Autodesk Fusion 360 part; units mm, degrees
sketch "Sketch1" plane through (0, 0, 0) normal (0, 0, 1) x (1, 0, 0)
  line L0 (0, 57.15) -> (0, 0)
  line L1 (101.6, 57.15) -> (130.175, 57.15)
  line L2 (130.175, 57.15) -> (130.175, 25.4)
  line L3 (130.175, 25.4) -> (101.6, 25.4)
  line L4 (101.6, 25.4) -> (101.6, 57.15)
  line L5 (115.8875, 25.4) -> (115.8875, 0) construction
  line L6 (106.3625, 25.4) -> (106.3625, 0)
  line L7 (125.4125, 25.4) -> (125.4125, 0)
  line L8 (12.7, 57.15) -> (12.7, 12.7)
  line L9 (12.7, 12.7) -> (28.575, 12.7)
  line L10 (28.575, 12.7) -> (28.575, 57.15)
  line L11 (14.2875, 12.7) -> (14.2875, 0)
  line L12 (26.9875, 12.7) -> (26.9875, 0)
  line L13 (12.7, 57.15) -> (28.575, 57.15)
  line L14 (14.2875, 0) -> (26.9875, 0)
  line L15 (106.3625, 0) -> (125.4125, 0)
  line L16 (36.5125, 0) -> (49.2125, 0)
  line L17 (34.925, 57.15) -> (50.8, 57.15)
  line L18 (49.2125, 12.7) -> (49.2125, 0)
  line L19 (34.925, 57.15) -> (34.925, 12.7)
  line L20 (36.5125, 12.7) -> (36.5125, 0)
  line L21 (34.925, 12.7) -> (50.8, 12.7)
  line L22 (50.8, 12.7) -> (50.8, 57.15)
  line L23 (58.7375, 0) -> (71.4375, 0)
  line L24 (57.15, 57.15) -> (73.025, 57.15)
  line L25 (71.4375, 12.7) -> (71.4375, 0)
  line L26 (57.15, 57.15) -> (57.15, 12.7)
  line L27 (58.7375, 12.7) -> (58.7375, 0)
  line L28 (57.15, 12.7) -> (73.025, 12.7)
  line L29 (73.025, 12.7) -> (73.025, 57.15)
  line L30 (80.9625, 0) -> (93.6625, 0)
  line L31 (79.375, 57.15) -> (95.25, 57.15)
  line L32 (93.6625, 12.7) -> (93.6625, 0)
  line L33 (79.375, 57.15) -> (79.375, 12.7)
  line L34 (80.9625, 12.7) -> (80.9625, 0)
  line L35 (79.375, 12.7) -> (95.25, 12.7)
  line L36 (95.25, 12.7) -> (95.25, 57.15)
  line L37 (141.2875, 25.4) -> (141.2875, 0)
  line L38 (136.525, 57.15) -> (165.1, 57.15)
  line L39 (150.8125, 25.4) -> (150.8125, 0) construction
  line L40 (136.525, 25.4) -> (136.525, 57.15)
  line L41 (165.1, 25.4) -> (136.525, 25.4)
  line L42 (165.1, 57.15) -> (165.1, 25.4)
  line L43 (160.3375, 25.4) -> (160.3375, 0)
  line L44 (141.2875, 0) -> (160.3375, 0)
  line L45 (176.2125, 25.4) -> (176.2125, 0)
  line L46 (171.45, 57.15) -> (200.025, 57.15)
  line L47 (185.7375, 25.4) -> (185.7375, 0) construction
  line L48 (171.45, 25.4) -> (171.45, 57.15)
  line L49 (200.025, 25.4) -> (171.45, 25.4)
  line L50 (200.025, 57.15) -> (200.025, 25.4)
  line L51 (195.2625, 25.4) -> (195.2625, 0)
  line L52 (176.2125, 0) -> (195.2625, 0)
  line L53 (211.1375, 25.4) -> (211.1375, 0)
  line L54 (206.375, 57.15) -> (234.95, 57.15)
  line L55 (220.6625, 25.4) -> (220.6625, 0) construction
  line L56 (206.375, 25.4) -> (206.375, 57.15)
  line L57 (234.95, 25.4) -> (206.375, 25.4)
  line L58 (234.95, 57.15) -> (234.95, 25.4)
  line L59 (230.1875, 25.4) -> (230.1875, 0)
  line L60 (211.1375, 0) -> (230.1875, 0)
  line L61 (317.5, 57.15) -> (317.5, 0)
  line L62 (317.5, 0) -> (0, 0)
  line L63 (317.5, 57.15) -> (0, 57.15)
  line L64 (265.1125, 25.4) -> (265.1125, 0)
  line L65 (241.3, 57.15) -> (269.875, 57.15)
  line L66 (255.5875, 25.4) -> (255.5875, 0) construction
  line L67 (246.0625, 25.4) -> (246.0625, 0)
  line L68 (269.875, 25.4) -> (241.3, 25.4)
  line L69 (246.0625, 0) -> (265.1125, 0)
  line L70 (269.875, 57.15) -> (269.875, 25.4)
  line L71 (241.3, 25.4) -> (241.3, 57.15)
  line L72 (300.0375, 25.4) -> (300.0375, 0)
  line L73 (276.225, 57.15) -> (304.8, 57.15)
  line L74 (290.5125, 25.4) -> (290.5125, 0) construction
  line L75 (280.9875, 25.4) -> (280.9875, 0)
  line L76 (304.8, 25.4) -> (276.225, 25.4)
  line L77 (280.9875, 0) -> (300.0375, 0)
  line L78 (304.8, 57.15) -> (304.8, 25.4)
  line L79 (276.225, 25.4) -> (276.225, 57.15)
  dimension "d2" = 57.15
  dimension "d4" = 28.575
  dimension "d6" = 9.525
  dimension "d7" = 9.525
  dimension "d21" = 15.875
  dimension "d23" = 12.7
  dimension "d24" = 1.5875
  dimension "d25" = 15.875
  dimension "d26" = 12.7
  dimension "d27" = 1.5875
  dimension "d28" = 15.875
  dimension "d29" = 12.7
  dimension "d30" = 1.5875
  dimension "d31" = 15.875
  dimension "d32" = 12.7
  dimension "d33" = 1.5875
  dimension "d34" = 6.35
  dimension "d35" = 6.35
  dimension "d36" = 6.35
  dimension "d37" = 12.7
  dimension "d38" = 6.35
  dimension "d39" = 31.75
  dimension "d40" = 28.575
  dimension "d41" = 9.525
  dimension "d42" = 9.525
  dimension "d43" = 31.75
  dimension "d44" = 28.575
  dimension "d45" = 9.525
  dimension "d46" = 9.525
  dimension "d47" = 31.75
  dimension "d48" = 28.575
  dimension "d49" = 9.525
  dimension "d50" = 9.525
  dimension "d51" = 31.75
  dimension "d52" = 6.35
  dimension "d53" = 6.35
  dimension "d54" = 6.35
  dimension "d56" = 28.575
  dimension "d57" = 9.525
  dimension "d58" = 9.525
  dimension "d59" = 31.75
  dimension "d60" = 28.575
  dimension "d61" = 9.525
  dimension "d62" = 9.525
  dimension "d63" = 31.75
  dimension "d64" = 6.35
  dimension "d65" = 6.35
  dimension "d66" = 12.7
extrude "Extrude3" add sketch "Sketch1" against normal blind 31.75
extrude "Extrude6" cut sketch "Sketch1" against normal blind 12.7 contours L1 L2 L3 L4 L63 | L3 L6 L7 L15 L62 | L38 L40 L41 L42 L63 | L37 L41 L43 L44 L62 | L46 L48 L49 L50 L63 | L45 L49 L51 L52 L62 | L54 L56 L57 L58 L63 | L53 L57 L59 L60 L62 | L63 L65 L68 L70 L71 | L62 L64 L67 L68 L69 | L63 L73 L76 L78 L79 | L62 L72 L75 L76 L77
extrude "Extrude7" cut sketch "Sketch1" against normal blind 12.7 contours L8 L9 L10 L13 L63 | L9 L11 L12 L14 L62 | L17 L19 L21 L22 L63 | L16 L18 L20 L21 L62 | L24 L26 L28 L29 L63 | L23 L25 L27 L28 L62 | L31 L33 L35 L36 L63 | L30 L32 L34 L35 L62
extrude "Extrude8" cut 4 faces at (77.2583, 4.2333, 0) (55.0333, 4.2333, 0) (32.8083, 4.2333, 0) (4.2333, 23.2833, 0) along direction (0, 0, -1) blind 6.35
equation "d21 = ( 5 / 8 ) * 1 in"
equation "d24 = ( 1 / 16 ) * 1 in"
equation "d25 = ( 5 / 8 ) * 1 in"
equation "d27 = ( 1 / 16 ) * 1 in"
equation "d28 = ( 5 / 8 ) * 1 in"
equation "d30 = ( 1 / 16 ) * 1 in"
equation "d31 = ( 5 / 8 ) * 1 in"
equation "d33 = ( 1 / 16 ) * 1 in"
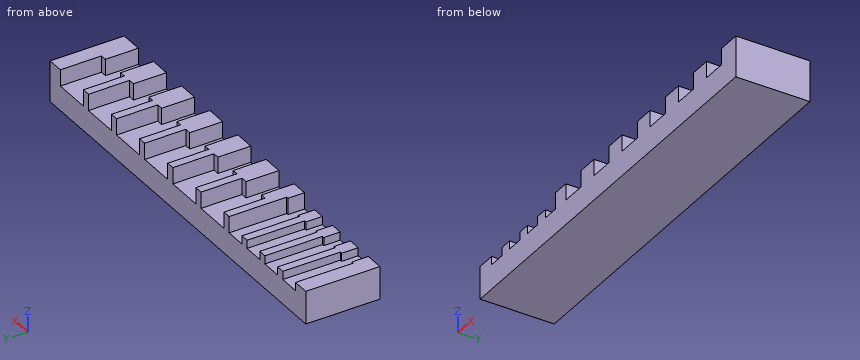
The listing builds one solid part. Answer for the finished solid, in the listing's coordinates (mm). Round coordinates to 2 decimals unless told otherwise and drop trailing zeros. Order: outer loops, then holes, each group sorted by start corner. A loop starts at its lowest first (then second) coordinate and runs counter-clockwise, first axis right, second up. Notation, with made-up numbers: (56.25, -2) - (81.25, -2) arc R14 ccw to (81.25, 18) - close; hole circle Ø10 at (-35.5, -40). An arc over 180 degrees is marked (long way). Write item = value, one per line. Start each with the question number.
1) Given pin 1 (1.7 mm diameter, centred on x = 28, z = -9, fed in from +Y); pin 2 (17.5 mm diameter, centred on x = 23.5, y = 39.5, fed in from +Z); pin 3 (1.4 mm diameter, centred on x = 197, z = -7.5, fed in from +Y), each flat-ended and moving along its own axis, determine where each tip first touches the part or whether it passes through.
2) Straight lines are drawn through the part: L1, parallel to Z at x = 33, y = 13.5; L2, parallel to Z at x = 26.5, y = 17; L3, parallel to Y at x = 230.5, z = -5. For each, find the intervals that lie inside material, in ascending order.
3) Section A-A, the plane z = -9.5 is taken. Count the separate pieces of the cut face and the enclosed holes in it, plus the area to 3 significant figures.
4) Section B-B, the plane x = 21.5 is taken. Write down the section's boundary in (y, z).
Results list:
q1.pin_1 = 57.15
q1.pin_2 = -6.35
q1.pin_3 = 25.4
q2.L1 = -31.75 to -6.35
q2.L2 = -31.75 to -12.7
q2.L3 = 0 to 25.4
q3.separate_pieces = 11
q3.enclosed_holes = 0
q3.area = 6,330 mm^2
q4.outline = (0, -31.75) - (57.15, -31.75) - (57.15, -12.7) - (0, -12.7) - close
